Answer from the drawing. Dimensions are ordinates in mm from the lowest x, y and z of the part. Give positions to 0.01 mm unless a question says otherwise; leave off trailing zeros. Write each loop counter-clockwise with the first axis right and the second up, starting at its lowest first coordinate (ties: lowest second). Pieces come first, ordered by that corner, then holes.
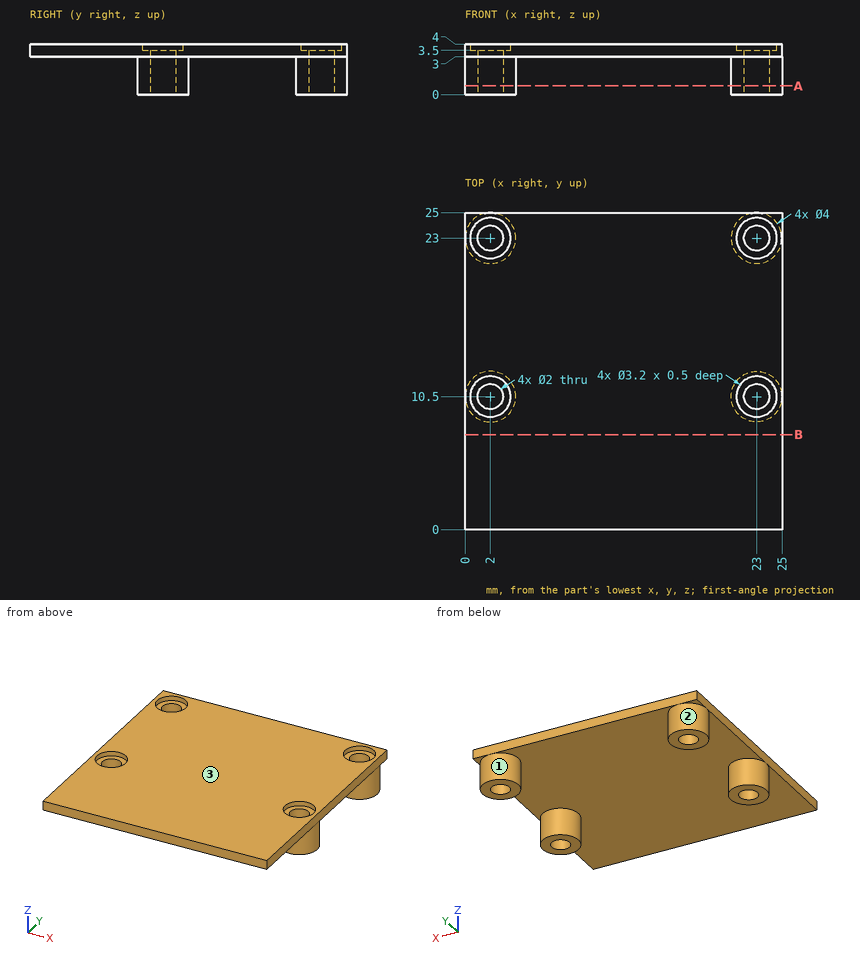
Item 1: Section A-A (z = 0.7) is taken. Write down the section's boundary in (x, y), and give its area (3 significant figures).
Result set:
outline: circle Ø4 at (2, 10.5); circle Ø4 at (2, 23); circle Ø4 at (23, 10.5); circle Ø4 at (23, 23); hole circle Ø2 at (2, 10.5); hole circle Ø2 at (2, 23); hole circle Ø2 at (23, 10.5); hole circle Ø2 at (23, 23)
area: 37.7 mm2
Item 2: Determine the mould class of the marked faces 1, 2 and 3 for opening direction Y: pulls with the +Y half, pulls with the -Y half, needs draft (parallel to the pull), parting line crosses it, or undercut.
Result set:
face 1: undercut
face 2: undercut
face 3: needs draft
Item 3: Section B-B (y = 7.5) is taken. Write down the section's boundary in (x, z).
Result set:
outline: (0, 3) - (25, 3) - (25, 4) - (0, 4) - close
Item 4: This flat-tipped pin is pushed along its axis until it touches: pin 1 Ø2.5 at (x, y) = (2, 10.5) entering from +Z. Where does it stop, or does it pass through?
Result set:
pin 1: stops at z = 3.5
Item 5: Find the intervals of material crossed by line 1 along X through (y, z) = (10.5, 3.7); line 2 along X through (y, z) = (23, 2.5); line 3 along Y through (x, z) = (2, 1.8), in increasing order.
Result set:
line 1: x = 0 to 0.4, 3.6 to 21.4, 24.6 to 25
line 2: x = 0 to 1, 3 to 4, 21 to 22, 24 to 25
line 3: y = 8.5 to 9.5, 11.5 to 12.5, 21 to 22, 24 to 25
